Part print with two shaded views. Sizes in mm from the minimum x, y, z corner. A direction names the side the tool comes from. Round coordinates to 2 decimals unless told otherwise and drop trailing zeros. Write each loop counter-clockwise with the first axis right and the second up, starting at its lowest first coordinate (ties: lowest second). Pieces come first, ordered by that corner, then holes. Notation, with made-up numbers: (78, 6.25) - (102, 6.25) arc R19 cw to (102, 15.25) - close; hole circle Ø10 at (61, -3). An arc over 180 degrees is marked (long way). Answer as a JSON object with one key per item and string values. Group by question number.
Item 1: Slice it at C-C, the plane z = 19. List the corners of the cut face in (x, y), then the cut area to 3 significant figures.
Item 2: Probe line 1 (Y direction, x = 13, z = 11); line 2 (Z direction, x = 25, y = 26); line 3 (Z direction, x = 50, y = 3.5). List the from-to ranges inside material, lowest first. Write a range as from..to.
Item 3: Slice it at B-B, the plane x = 11. List the corners of the cut face in (y, z), then the cut area to 4 significant figures.
Item 4: Slice it at A-A, the plane y = 24. List the corners of the cut face in (x, z), then the cut area to 4 significant figures.
Item 5: Slice it at D-D, the plane z = 49. List the corners of the cut face in (x, y), then the cut area to 3 significant figures.
Item 6: Two-plate mould, pull along Y, no slides. Class the marked faces 1, 2, 3 and 4: +Y half, -Y half, draft (parallel to the pull), parting line (faces both ways), or undercut.
Item 7: Flat gauge pins, fed straight in: pin 1 (8 mm diameter, centred on y = 25.5, z = 51, fed in from -X); pin 2 (3 mm diameter, centred on x = 11, z = 51.5, fed in from -Y); pin 3 (3 mm diameter, centred on x = 37.5, z = 49.5, fed in from -Y); pin 4 (5 mm diameter, centred on y = 42, z = 39, fed in from -X). Where does each tip first touch, or does it go through?
Item 8: Which spindle directions (+Z, -Z, +X, -X, +Y, -Y) get a long thin tool onto all of the face, cutting with end or side? Do the marked faces 5, 6, 7, 8 and 9. Say none if no direction does.
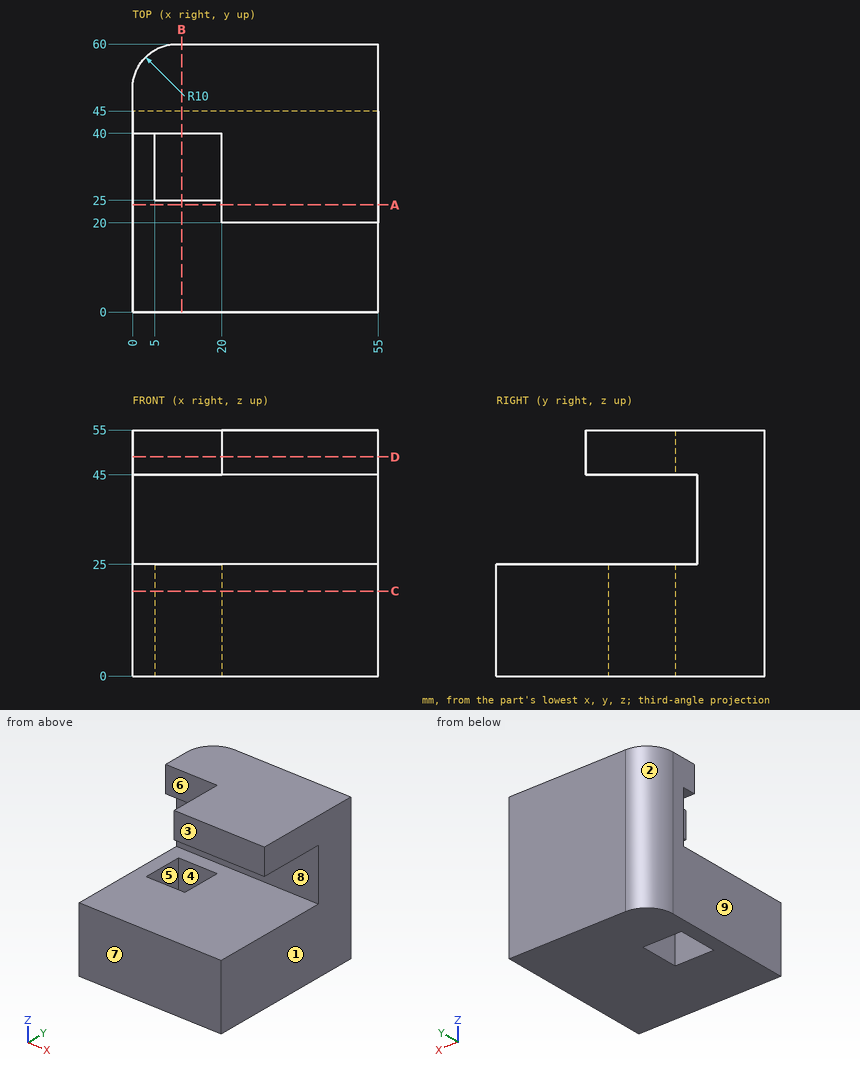
Geometry says:
{
 "1": {"outline": "(0, 0) - (55, 0) - (55, 60) - (10, 60) arc R10 ccw to (0, 50) - close; hole (5, 25) - (20, 25) - (20, 40) - (5, 40) - close", "area": "3,050 mm^2"},
 "2": {"line 1": "y = 0..25, 40..60", "line 2": "z = 0..25, 45..55", "line 3": "z = 0..25"},
 "3": {"outline": "(0, 0) - (25, 0) - (25, 25) - (0, 25) - close; (40, 0) - (60, 0) - (60, 55) - (40, 55) - (40, 45) - (45, 45) - (45, 25) - (40, 25) - close", "area": "1,625 mm^2"},
 "4": {"outline": "(0, 0) - (55, 0) - (55, 25) - (0, 25) - close; (20, 45) - (55, 45) - (55, 55) - (20, 55) - close", "area": "1,725 mm^2"},
 "5": {"outline": "(0, 40) - (20, 40) - (20, 20) - (55, 20) - (55, 60) - (10, 60) arc R10 ccw to (0, 50) - close", "area": "1,780 mm^2"},
 "6": {"face 1": "draft", "face 2": "+Y half", "face 3": "-Y half", "face 4": "undercut"},
 "7": {"pin 1": "stops at x = 20", "pin 2": "stops at y = 40", "pin 3": "stops at y = 20", "pin 4": "passes through"},
 "8": {"face 5": "+Z, -Z", "face 6": "+Z, -X, -Y", "face 7": "+Z, -Z, +X, -X, -Y", "face 8": "+X, -X, -Y", "face 9": "+Z, -Z, -X, +Y, -Y"}
}
